Here's how the part is built. I have some questions about the finished solid (model axes, mm). A direction names the side the tool comes from. Coordinates: 2 decimals unless noted, no trailing zeros. Write each loop counter-clockwise with the first axis right and the second up, starting at its lowest first coordinate (ties: lowest second). Pieces come first, ordered by that corner, then holes. Notation, with made-up numbers: (-27, -30.5) -> (-14, -30.5) arc R5 cw to (-14, -25.5) -> close; hole circle Ø6 at (79, 75.5). An arc over 180 degrees is marked (long way). Use a Markdown table: item, result. Add a question column.
Item 1: If I drill on line 1 along X through (y, z) = (-4.5, 0.45); line 2 along X through (y, z) = (-5.5, -1.2); line 3 along X through (y, z) = (-20, -0.4), over which ranges is the centre line in solid material (lowest first)? Write a range as from..to.
Item 2: Imagine slicing it at C-C, the plane x = -11.5. Write out the boundary of the cut face in (y, z).
Item 3: Imagine slicing it at B-B, the plane z = -0.5. Count the separate pieces of the cut face and the enclosed holes in it, and give its area (3 significant figures).
Item 4: On a 3-axis mill with a long thin cutter (end or side, diameter ignored), from which of +Z, -Z, +X, -X, +Y, -Y can I reach the whole of each face in a straight line? I mean faces 1 (the cylindrical face through (-0.704, -14.821, 0.021)), 2 (the cylindrical face through (21.941, 3.024, 0.021)), 3 (the flat face through (11, -5, 1.5)). Say none if no direction works.
Item 5: Imagine slicing it at D-D, the plane x = 30. Write out the boundary of the cut face in (y, z).
Item 6: Imagine slicing it at A-A, the plane x = 60. Write out the boundary of the cut face in (y, z), and give its area (3 significant figures).
Item 7: Will this pin go through, and if not, where does the flat tip stop? pin 1 Ø1 at (x, z) = (8, 0) entering from -Y.
```python
from build123d import *

# Parameters (mm, degrees)
EXTRUDE_1_DEPTH          = 1.5
CUT_EXTRUDE_1_DEPTH      = 2.5
CUT_EXTRUDE_1_DEPTH_BACK = 2.5
FILLET_2_R               = 0.5
SKETCH_1_3_R             = 2.55
CUT_EXTRUDE_2_DEPTH      = 2.5000001
CUT_EXTRUDE_2_DEPTH_BACK = 2.5000001
FILLET_3_R               = 1
FILLET_4_R               = 6


with BuildPart() as part:
    # 草图3 → 凸台-拉伸1 (new body, symmetric)
    with BuildSketch(Plane.XY):
        with BuildLine():
            Line((-69, 0.053699407), (-17.857896917, 2.8))
            ThreePointArc((-17.857896917, 2.8), (-12.910589699, 3.119021237), (-8, 3.8))
            ThreePointArc((-8, 3.8), (-2.43432215, 6.908286356), (0, 12.8))
            Line((0, 12.8), (4, 12.8))
            ThreePointArc((4, 12.8), (8.414270073, 5.897124087), (16, 2.8))
            ThreePointArc((16, 2.8), (17, 2.759720994), (18, 2.8))
            ThreePointArc((18, 2.8), (21.996883494, 3.025702827), (26, 3.058530741))
            ThreePointArc((26, 3.058530741), (52.423511602, 2.290913304), (78.817734107, 0.82933187))
            ThreePointArc((78.817734107, 0.82933187), (86.700158242, -2.881010306), (89.995283198, -10.945835216))
            ThreePointArc((89.995283198, -10.945835216), (89.543787999, -17.161843843), (88, -23.2))
            Line((88, -23.2), (82, -23.2))
            ThreePointArc((82, -23.2), (78.162031949, -17.126267779), (71.242138758, -15.193575339))
            ThreePointArc((71.242138758, -15.193575339), (60.309670553, -15.485417284), (49.439553231, -14.283509554))
            ThreePointArc((49.439553231, -14.283509554), (28.723471343, -12.408337394), (8, -14.2))
            ThreePointArc((8, -14.2), (2.43432215, -17.308286356), (0, -23.2))
            Line((0, -23.2), (-4, -23.2))
            ThreePointArc((-4, -23.2), (-8.414270073, -16.297124087), (-16, -13.2))
            ThreePointArc((-16, -13.2), (-37.993667939, -11.512934158), (-60, -10))
            Line((-60, -10), (-70, 0))
            Line((-70, 0), (-69, 0.053699407))
        make_face()
    extrude(amount=EXTRUDE_1_DEPTH, both=True)

    # 草图1 → 切除-拉伸1 (cut, two sides)
    with BuildSketch(Plane.XY) as cut_extrude_1_sk:
        with BuildLine():
            ThreePointArc((10.342236489, 0.104989325), (5.407803908, -0.918324974), (0.762235002, 1.034746091))
            ThreePointArc((0.762235002, 1.034746091), (-0.220251061, 1.823323048), (-1.237764998, 2.566154029))
            ThreePointArc((-1.237764998, 2.566154029), (0.767930164, 4.495803013), (2.342236489, 6.790997533))
            ThreePointArc((2.342236489, 6.790997533), (5.834327754, 2.840266104), (10.342236489, 0.104989325))
        make_face()
        with BuildLine():
            ThreePointArc((-0.762235002, -11.434746091), (0.220251061, -12.223323048), (1.237764998, -12.966154029))
            ThreePointArc((1.237764998, -12.966154029), (-0.767930164, -14.895803013), (-2.342236489, -17.190997533))
            ThreePointArc((-2.342236489, -17.190997533), (-5.834327754, -13.240266104), (-10.342236489, -10.504989325))
            ThreePointArc((-10.342236489, -10.504989325), (-5.407803908, -9.481675026), (-0.762235002, -11.434746091))
        make_face()
    extrude(amount=CUT_EXTRUDE_1_DEPTH, mode=Mode.SUBTRACT)
    extrude(cut_extrude_1_sk.sketch, amount=-CUT_EXTRUDE_1_DEPTH_BACK, mode=Mode.SUBTRACT)

    # 圆角2
    fillet_2_edges = [part.edges().sort_by_distance(p)[0] for p in [
        (10.342236489, 0.104989325, 0),
        (-1.237764998, 2.566154029, 0),
        (2.342236489, 6.790997533, 0),
        (1.237764998, -12.966154029, 0),
        (-2.342236489, -17.190997533, 0),
        (-10.342236489, -10.504989325, 0),
    ]]
    fillet(fillet_2_edges, radius=FILLET_2_R)

    # 草图1<3> → 切除-拉伸2 (cut, two sides)
    with BuildSketch(Plane.XY) as cut_extrude_2_sk:
        with Locations((60, -6.8)):
            Circle(SKETCH_1_3_R)
        with Locations((26, -4.5)):
            Circle(SKETCH_1_3_R)
    extrude(amount=CUT_EXTRUDE_2_DEPTH, mode=Mode.SUBTRACT)
    extrude(cut_extrude_2_sk.sketch, amount=-CUT_EXTRUDE_2_DEPTH_BACK, mode=Mode.SUBTRACT)

    # 圆角3
    fillet_3_edges = [part.edges().sort_by_distance(p)[0] for p in [
        (0, 12.8, 0),
        (4, 12.8, 0),
        (82, -23.2, 0),
        (0, -23.2, 0),
        (-4, -23.2, 0),
    ]]
    fillet(fillet_3_edges, radius=FILLET_3_R)

    # 圆角4
    fillet_4_edges = [part.edges().sort_by_distance(p)[0] for p in [
        (88, -23.2, 0),
    ]]
    fillet(fillet_4_edges, radius=FILLET_4_R)


solid = part.part
```
Ans:
| question | item | result |
|---|---|---|
| 1 | line 1 | x = -65.5..23.45, 28.55..58.9, 61.1..87.99 |
| 1 | line 2 | x = -64.5..23.65, 28.35..57.81, 62.19..88.59 |
| 1 | line 3 | x = -5.31..0.74, 80.76..88.75 |
| 2 | outline | (-14.36, -1.5) -> (3.28, -1.5) -> (3.28, 1.5) -> (-14.36, 1.5) -> close |
| 3 | separate pieces | 1 |
| 3 | enclosed holes | 4 |
| 3 | area | 2,480 mm^2 |
| 4 | face 1 | +Z, -Z |
| 4 | face 2 | +Z, -Z, +Y |
| 4 | face 3 | +Z, +X, -X, +Y, -Y |
| 5 | outline | (-12.42, -1.5) -> (2.99, -1.5) -> (2.99, 1.5) -> (-12.42, 1.5) -> close |
| 6 | outline | (-15.47, -1.5) -> (-9.35, -1.5) -> (-9.35, 1.5) -> (-15.47, 1.5) -> close; (-4.25, -1.5) -> (1.94, -1.5) -> (1.94, 1.5) -> (-4.25, 1.5) -> close |
| 6 | area | 36.9 mm^2 |
| 7 | pin 1 | stops at y = -14.3 |
